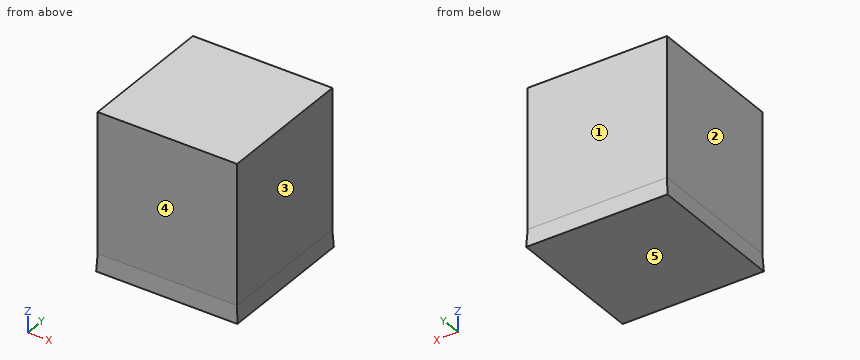
```python
from build123d import *

# Parameters (mm, degrees)
F0_W     = 25.4
F0_H     = 25.4
F1_DEPTH = 3.175
F1_TAPER = -3
F2_DEPTH = 25.4


with BuildPart() as f1:
    # F0 (on Top) → F1 (new body)
    with BuildSketch(Plane.XY):
        Rectangle(F0_W, F0_H)
    extrude(amount=-F1_DEPTH, taper=F1_TAPER)

    # F2 (add): a face of the model
    f2_faces = [f1.faces().sort_by_distance(p)[0] for p in [
        (0, 0, 0),
    ]]
    extrude(f2_faces, amount=F2_DEPTH)


solid = f1.part
```
Part model, mm, in its own coordinate system. Face numbers are marked on the shaded views. A direction names the side the tool comes from. Round coordinates to 2 decimals unless told otherwise and drop trailing zeros. Write each loop counter-clockwise with the first axis right and the second up, starting at its lowest first coordinate (ties: lowest second). Pieces come first, ordered by that corner, then holes. Notation, with made-up numbers: (-2.5, 13.25) -> (23.5, 13.25) arc R18 cw to (23.5, 26.25) -> close; hole circle Ø4 at (70.25, 81.25). An arc over 180 degrees is marked (long way). Return JSON: item names as keys, results as strings. Group by question number.
Q1. Probe L1, parallel to Y at x = 10, z = 0.5. List the from-to ranges inside material, lowest first. Write a range as [from, to].
Q2. Mould opens along X. For the marked faces 1, 2 and 3 say: pulls with the +X half, pulls with the -X half, needs draft (parallel to the pull), parting line crosses it, or undercut.
Q3. Pin check, flat tips, straight feed: pin 1 (2 mm diameter, centred on x = 0.5, z = 9.5, fed in from +Y); pin 2 (1 mm diameter, centred on y = -6, z = 11.5, fed in from -X); pin 3 (1.5 mm diameter, centred on x = -7.5, z = 4.5, fed in from -Y). Stop position of each tip, or through.
Q4. Saw through at A-A on z = 14.5. Write the cut outline in (x, y), plus the area to 3 significant figures.
Q5. Which spindle directions (+Z, -Z, +X, -X, +Y, -Y) get a long thin tool onto all of the face, cutting with end or side? Do the marked faces 4 and 5. Say none if no direction does.
Answer:
{
 "1": {"L1": "[-12.7, 12.7]"},
 "2": {"face 1": "needs draft", "face 2": "pulls with the -X half", "face 3": "pulls with the +X half"},
 "3": {"pin 1": "y = 12.7", "pin 2": "x = -12.7", "pin 3": "y = -12.7"},
 "4": {"outline": "(-12.7, -12.7) -> (12.7, -12.7) -> (12.7, 12.7) -> (-12.7, 12.7) -> close", "area": "645 mm2"},
 "5": {"face 4": "+Z, +X, -X, -Y", "face 5": "-Z, +X, -X, +Y, -Y"}
}
